Model file for the job. Use its own axes, mm. Face numbers are marked on the shaded views. A direction names the side the tool comes from. Coordinates: 2 decimals unless noted, no trailing zeros. Loops run counter-clockwise (first coordinate to the right, second up) from the corner with the lowest first, then second, coordinate; pieces in that order, holes last.
from build123d import *

# Parameters (mm, degrees)
F0_R     = 1.55
F0_R_2   = 10
F1_DEPTH = 25


with BuildPart() as f1:
    # F0 (on Front) → F1 (new body)
    with BuildSketch(Plane.XZ):
        with BuildLine():
            Line((52, 21.25), (0, 21.25))
            ThreePointArc((0, 21.25), (15.026019, 15.026019), (21.25, 0))
            ThreePointArc((21.25, 0), (15.026019, -15.026019), (0, -21.25))
            Line((0, -21.25), (52, -21.25))
            ThreePointArc((52, -21.25), (54.12132, -20.37132), (55, -18.25))
            Line((55, -18.25), (55, 18.25))
            ThreePointArc((55, 18.25), (54.12132, 20.37132), (52, 21.25))
        make_face()
        with BuildLine():
            Line((45, -13), (30, -13))
            ThreePointArc((30, -13), (27, -10), (30, -7))
            Line((30, -7), (45, -7))
            ThreePointArc((45, -7), (48, -10), (45, -13))
        make_face(mode=Mode.SUBTRACT)
        with BuildLine():
            Line((45, 7), (30, 7))
            ThreePointArc((30, 7), (27, 10), (30, 13))
            Line((30, 13), (45, 13))
            ThreePointArc((45, 13), (48, 10), (45, 7))
        make_face(mode=Mode.SUBTRACT)
        with BuildLine():
            ThreePointArc((21.25, 0), (15.026019, 15.026019), (0, 21.25))
            ThreePointArc((0, 21.25), (-21.25, 0), (0, -21.25))
            ThreePointArc((0, -21.25), (15.026019, -15.026019), (21.25, 0))
        make_face()
        with Locations((-12.990381, -7.5)):
            Circle(F0_R, mode=Mode.SUBTRACT)
        with Locations((12.990381, -7.5)):
            Circle(F0_R, mode=Mode.SUBTRACT)
        Circle(F0_R_2, mode=Mode.SUBTRACT)
        with Locations((0, 15)):
            Circle(F0_R, mode=Mode.SUBTRACT)
    extrude(amount=F1_DEPTH)


solid = f1.part
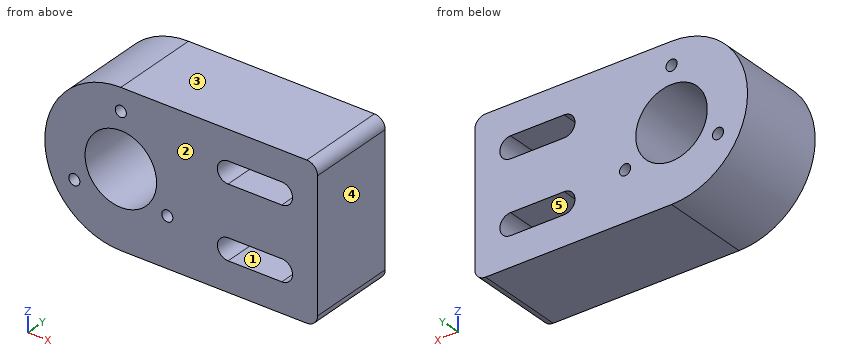
Q1. Mould opens along Z. For the marked faces 3, 4 and 5 say: +Z half, -Z half, draft (parallel to the pull), parting line (faces both ways), or undercut.
Answers:
face 3: +Z half
face 4: draft
face 5: undercut
Q2. Slice it at C-C (y = -23). List the corners of the cut face in (x, z).
Answers:
outline: (0, -21.25) - (52, -21.25) arc R3 ccw to (55, -18.25) - (55, 18.25) arc R3 ccw to (52, 21.25) - (0, 21.25) arc R21.25 ccw to start; hole circle Ø3.1 at (-12.99, -7.5); hole circle Ø20 at (0, 0); hole circle Ø3.1 at (0, 15); hole circle Ø3.1 at (12.99, -7.5); hole (30, -13) - (45, -13) arc R3 ccw to (45, -7) - (30, -7) arc R3 ccw to start; hole (30, 7) - (45, 7) arc R3 ccw to (45, 13) - (30, 13) arc R3 ccw to start
Q3. Which spindle directions (+Z, -Z, +X, -X, +Y, -Y) get a long thin tool onto all of the face, cutting with end or side? Do the marked faces 1 and 2. Say none if no direction does.
Answers:
face 1: +Y, -Y
face 2: +Z, -Z, +X, -X, -Y
Q4. Drill centre lines: line 1 (Z direction, x = 34.5, y = -7.75); line 2 (X direction, y = -20.5, z = -8); line 3 (Z direction, x = 13, y = -5). Where is each one in solid material? Low to high.
Answers:
line 1: z = -21.25 to -13, -7 to 7, 13 to 21.25
line 2: x = -19.69 to -14.46, -11.52 to -6, 6 to 11.52, 14.46 to 27.76, 47.24 to 55
line 3: z = -21.25 to -9.05, -5.95 to 21.25
Q5. Slice it at B-B (x = 3). List the corners of the cut face in (y, z).
Answers:
outline: (-25, -21.25) - (0, -21.25) - (0, -9.54) - (-25, -9.54) - close; (-25, 9.54) - (0, 9.54) - (0, 21.25) - (-25, 21.25) - close
Q6. Flat gauge pins, fed straight in: P1, Ø2, axis at y = -3, z = 9, coming from the -X side; P2, Ø3, axis at x = -12.99, z = -7.5, coming from the +Y side; P3, Ø8, axis at x = -6.5, y = -20, coming from the +Z side. Where does each tip first touch, or does it go through?
Answers:
P1: stops at x = -19.69
P2: passes through
P3: stops at z = 21.1
Q7. Slice it at A-A (z = 0). List the corners of the cut face in (x, y), and give its area (3 significant figures).
Answers:
outline: (-21.25, -25) - (-10, -25) - (-10, 0) - (-21.25, 0) - close; (10, -25) - (55, -25) - (55, 0) - (10, 0) - close
area: 1,410 mm2
